from build123d import *

# Parameters (mm, degrees)
BOSS_EXTRUDE5_DEPTH   = 90
SKETCH11_3_R          = 55
BOSS_EXTRUDE6_DEPTH   = 115
SKETCH11_4_R          = 55
BOSS_EXTRUDE7_DEPTH   = 105
BOSS_EXTRUDE8_DEPTH   = 15
SKETCH17_R            = 45
BOSS_EXTRUDE9_DEPTH   = 80
SKETCH18_R            = 52
BOSS_EXTRUDE10_DEPTH  = 5
SKETCH19_R            = 27.5
SKETCH19_R_2          = 18
BOSS_EXTRUDE12_DEPTH  = 15
BODY_MOVE_COPY2_ANGLE = 180
SKETCH28_R            = 52
CUT_EXTRUDE2_DEPTH    = 60
CUT_EXTRUDE3_DEPTH    = 80
SKETCH31_R            = 30
CUT_EXTRUDE6_DEPTH    = 196
BODY_MOVE_COPY3_ANGLE = 180
BODY_MOVE_COPY4_ANGLE = 90
BODY_MOVE_COPY6_ANGLE = 180
BODY_MOVE_COPY8_ANGLE = 90
BODY_MOVE_COPY9_ANGLE = 90
SKETCH36_R            = 24.5
CUT_EXTRUDE7_DEPTH    = 60


with BuildPart() as part:
    # Sketch11 → Boss-Extrude5 (new body)
    with BuildSketch(Plane.XY):
        with BuildLine():
            Line((-45, 408.377223398), (-45, 31.622776602))
            ThreePointArc((-45, 31.622776602), (0, -55), (45, 31.622776602))
            Line((45, 31.622776602), (45, 408.377223398))
            ThreePointArc((45, 408.377223398), (0, 495), (-45, 408.377223398))
        make_face()
    extrude(amount=BOSS_EXTRUDE5_DEPTH)

    # Sketch11<3> → Boss-Extrude6 (add)
    with BuildSketch(Plane.XY):
        with Locations((0, 440)):
            Circle(SKETCH11_3_R)
    extrude(amount=BOSS_EXTRUDE6_DEPTH)

    # Sketch11<4> → Boss-Extrude7 (add)
    with BuildSketch(Plane.XY):
        Circle(SKETCH11_4_R)
    extrude(amount=BOSS_EXTRUDE7_DEPTH)

    # Sketch13 → Boss-Extrude8 (add)
    with BuildSketch(Plane.XY.offset(90)):
        with BuildLine():
            Line((7.638888889, 82), (7.638888889, 54.46693838))
            Line((7.638888889, 54.46693838), (-7.638888889, 54.46693838))
            Line((-7.638888889, 54.46693838), (-7.638888889, 82))
            ThreePointArc((-7.638888889, 82), (0, 89.638888889), (7.638888889, 82))
        make_face()
    extrude(amount=BOSS_EXTRUDE8_DEPTH)

    # Sketch17 → Boss-Extrude9 (add)
    with BuildSketch(Plane.XY.offset(115)):
        with Locations((0, 440)):
            Circle(SKETCH17_R)
    extrude(amount=BOSS_EXTRUDE9_DEPTH)

    # Sketch18 → Boss-Extrude10 (add)
    with BuildSketch(Plane(origin=(0, 0, 0), x_dir=(-1, 0, 0), z_dir=(0, 0, -1))):
        with Locations((0, 440)):
            Circle(SKETCH18_R)
    extrude(amount=BOSS_EXTRUDE10_DEPTH)

    # Sketch19 → Boss-Extrude12 (add)
    with BuildSketch(Plane(origin=(0, 0, -5), x_dir=(-1, 0, 0), z_dir=(0, 0, -1))):
        with Locations((0, 440)):
            Circle(SKETCH19_R)
        with Locations((0, 440)):
            Circle(SKETCH19_R_2, mode=Mode.SUBTRACT)
    extrude(amount=BOSS_EXTRUDE12_DEPTH)


with BuildPart() as part_1:
    # Body-Move/Copy2: moved
    add(part.part.rotate(Axis((0, 0, 0), (0, 1, 0)), BODY_MOVE_COPY2_ANGLE))

    # Sketch28 → Cut-Extrude2 (cut)
    with BuildSketch(Plane(origin=(0, 0, -105), x_dir=(-1, 0, 0), z_dir=(0, 0, -1))):
        Circle(SKETCH28_R)
    extrude(amount=-CUT_EXTRUDE2_DEPTH, mode=Mode.SUBTRACT)

    # Sketch29 → Cut-Extrude3 (cut)
    with BuildSketch(Plane.XY):
        with BuildLine():
            ThreePointArc((-30, 361), (-28.535533906, 364.535533906), (-25, 366))
            Line((-25, 366), (25, 366))
            ThreePointArc((25, 366), (28.535533906, 364.535533906), (30, 361))
            Line((30, 361), (30, 255))
            ThreePointArc((30, 255), (28.535533906, 251.464466094), (25, 250))
            Line((25, 250), (-25, 250))
            ThreePointArc((-25, 250), (-28.535533906, 251.464466094), (-30, 255))
            Line((-30, 255), (-30, 361))
        make_face()
        with BuildLine():
            ThreePointArc((-30, 185), (-28.535533906, 188.535533906), (-25, 190))
            Line((-25, 190), (25, 190))
            ThreePointArc((25, 190), (28.535533906, 188.535533906), (30, 185))
            Line((30, 185), (30, 79))
            ThreePointArc((30, 79), (28.535533906, 75.464466094), (25, 74))
            Line((25, 74), (-25, 74))
            ThreePointArc((-25, 74), (-28.535533906, 75.464466094), (-30, 79))
            Line((-30, 79), (-30, 185))
        make_face()
    extrude(amount=-CUT_EXTRUDE3_DEPTH, mode=Mode.SUBTRACT)

    # Sketch31 → Cut-Extrude6 (cut, through all)
    with BuildSketch(Plane.XY):
        Circle(SKETCH31_R)
    extrude(amount=-CUT_EXTRUDE6_DEPTH, mode=Mode.SUBTRACT)


with BuildPart() as part_2:
    # Body-Move/Copy3: moved
    add(part_1.part.moved(Location((0, 0, 0))).rotate(Axis((0, 0, -87.5), (0, 1, 0)), BODY_MOVE_COPY3_ANGLE))


with BuildPart() as part_3:
    # Body-Move/Copy4: moved
    add(part_2.part.rotate(Axis((0, 225, 0), (0, 0, -1)), BODY_MOVE_COPY4_ANGLE))


with BuildPart() as part_4:
    # Body-Move/Copy6: moved
    add(part_3.part.rotate(Axis((225, 0, -17.5), (0, 1, 0)), BODY_MOVE_COPY6_ANGLE))


with BuildPart() as part_5:
    # Body-Move/Copy7: moved
    add(part_4.part.moved(Location((-675, -225, -35))))


with BuildPart() as part_6:
    # Body-Move/Copy8: moved
    add(part_5.part.rotate(Axis((-225, 0, 0), (0, 0, -1)), BODY_MOVE_COPY8_ANGLE))


with BuildPart() as part_7:
    # Body-Move/Copy9: moved
    add(part_6.part.rotate(Axis((-225, 0, 0), (0, 0, -1)), BODY_MOVE_COPY9_ANGLE))


with BuildPart() as part_8:
    # Body-Move/Copy10: moved
    add(part_7.part.moved(Location((450, 1e-09, 0))))


with BuildPart() as part_9:
    # Body-Move/Copy14: moved
    add(part_8.part.moved(Location((0, 0, 62.63))))

    # Sketch36 → Cut-Extrude7 (cut)
    with BuildSketch(Plane(origin=(0, 0, -27.37), x_dir=(-1, 0, 0), z_dir=(0, 0, -1))):
        with Locations((-440, 2e-09)):
            Circle(SKETCH36_R)
    extrude(amount=-CUT_EXTRUDE7_DEPTH, mode=Mode.SUBTRACT)


solid = part_9.part
The listing builds one solid part. Answer for the finished solid, in the listing's coordinates (mm). A direction names the side the tool comes from. Coordinates: 2 decimals unless noted, no trailing zeros. Write each loop counter-clockwise with the first axis right and the second up, starting at its lowest first coordinate (ties: lowest second). Pieces come first, ordered by that corner, then holes. Notation, with made-up numbers: M 47.5,-16 L 79.5,-16 A21 cw 79.5,-10 Z; hole C -9,-39 d4. An arc over 180 degrees is marked long. Use one line per item in the form item = value.
Item 1: Find section D-D, the plane y = 35. Give the vertices of the cut face in (x, z), plus the area to 3 significant figures.
Model answer:
outline = M -42.43,62.63 L -38.46,62.63 L -38.46,122.63 L 38.46,122.63 L 38.46,62.63 L 42.43,62.63 L 42.43,77.63 L 397.57,77.63 L 397.57,52.63 L 411.72,52.63 L 411.72,-27.37 L 468.28,-27.37 L 468.28,52.63 L 482.43,52.63 L 482.43,167.63 L 478.46,167.63 L 478.46,172.63 L 401.54,172.63 L 401.54,167.63 L -42.43,167.63 Z
area = 50,900 mm2
Item 2: For faces 1 (the face through (50, -16, 62.63)), 2 (the face through (-22, 22, 122.63)), 3 (the face through (217, 45, 123)), 4 (the face through (418, -22, 172.63)), 5 (the face through (25.296, -16.128, 145.445)), determine the directions among +Z, -Z, +X, -X, +Y, -Y from which every point of the face is accessible in a straight line to the end or side of a thin tool.
Model answer:
face_1 = -Z, -X, +Y, -Y
face_2 = -Z
face_3 = +Z, -Z, +Y
face_4 = +Z
face_5 = +Z, -Z
Item 3: Find section A-A, the plane z = 110. Give the vertices of the cut face in (x, y).
Model answer:
outline = M 31.62,-45 L 408.38,-45 A55 ccw long 408.38,45 L 31.62,45 A55 ccw long Z; hole C 0,0 d104; hole M 74,-25 A5 ccw 79,-30 L 185,-30 A5 ccw 190,-25 L 190,25 A5 ccw 185,30 L 79,30 A5 ccw 74,25 Z; hole M 250,-25 A5 ccw 255,-30 L 361,-30 A5 ccw 366,-25 L 366,25 A5 ccw 361,30 L 255,30 A5 ccw 250,25 Z
Item 4: Find section C-C, the plane x = 267. Give the vertices of the cut face in (y, z), plus the area to 3 significant figures.
Model answer:
outline = M -45,77.63 L 45,77.63 L 45,167.63 L 30,167.63 L 30,87.63 L -30,87.63 L -30,167.63 L -45,167.63 Z
area = 3,300 mm2
Item 5: Given P1, Ø4, axis at x = 369.5, y = 42.5, coming from the +Z side; P2, Ø12, axis at x = 329, z = 102.5, coming from the -Y side; P3, Ø4, axis at y = -8.5, z = 135.5, coming from the +X side, each flat-ended and moving along its own axis, determine where each tip first touches the part or whether it passes through.
Model answer:
P1 = 167.63
P2 = -45
P3 = 494.61
Item 6: Find the intervals of material crossed by probe 1 along X at (y, z) = (1, 89.5); probe 2 along X at (y, z) = (0, 143); probe 3 along Y at (x, z) = (325.5, 135.5), in increasing order.
Model answer:
probe_1 = -54.99 to -51.99, 51.99 to 74, 190 to 250, 366 to 494.99
probe_2 = -55 to -30, 30 to 74, 190 to 250, 366 to 495
probe_3 = -45 to -30, 30 to 45
Item 7: The mould has two halves that part along X. Classify faces 6 (the face through (68, 7.639, 70)), 7 (the face through (389.237, 11.273, 170.095)), 8 (the face through (400, -21, 52.63)): released by +X, released by -X, zero draft, split by the parting line, or undercut.
Model answer:
face_6 = undercut
face_7 = split by the parting line
face_8 = zero draft
Item 8: Find section B-B, the plane x = -14.5. Give the vertices of the cut face in (y, z), plus the area to 3 significant figures.
Model answer:
outline = M -53.05,62.63 L -49.94,62.63 L -49.94,122.63 L -26.26,122.63 L -26.26,167.63 L -53.05,167.63 Z; M 26.26,122.63 L 49.94,122.63 L 49.94,62.63 L 53.05,62.63 L 53.05,167.63 L 26.26,167.63 Z
area = 2,790 mm2
